For this review, take the finished solid that the model builds, in its own axes (mm). A direction names the side the tool comes from. Give positions to 0.01 mm unless a question says otherwise; leave off trailing zeros. Loops run counter-clockwise (first coordinate to the right, second up) from the corner with the lowest first, then second, coordinate; pieces in that order, holes last. Notation, with made-up numbers: (30.25, 55) - (89.25, 55) arc R20 ccw to (89.25, 67) - close; hole circle Ø9 at (39, 21.5). An arc over 180 degrees is marked (long way). Use CSV: the item, a comma, the result in double quotes. Start each with the question number.
1. For pin 1 (1 mm diameter, centred on x = 765, y = 14, fed in from +Z); pin 2 (9.5 mm diameter, centred on x = 750, y = 29.31, fed in from +Z) (1 decimal); pin 3 (8.5 mm diameter, centred on x = 755.5, y = 37, fed in from -Z); pin 4 (1 mm diameter, centred on x = 767, z = -4, fed in from -Y), all flat-tipped, find the tip position at first contact; note any pin that passes through.
2. Mouldability with a two-part tool opening along Y and no side actions: class faces 1 (the flat face through (750, 15, -10)), 2 (the flat face through (745, 40, 1)) as pulls with the +Y half, pulls with the -Y half, needs draft (parallel to the pull), parting line crosses it, or undercut.
3. For faces 3 (the flat face through (755, 40, 1)), 4 (the flat face through (750, 20, -1)), 5 (the flat face through (750, 20, 3)), list the 3-axis set-ups (+Z, -Z, +X, -X, +Y, -Y) from which the entire face can be reached by the end or side of a thin tool; tool diameter is ignored.
4. Take a section at B-B on x = 750. Give the boundary of the cut face in (y, z), plus the area to 3 significant figures.
5. Take a section at A-A on z = -5. State how many separate pieces and enclosed holes the cut face has, plus the area to 3 significant figures.
6. Wall thickness on line 1 (Y direction, x = 750, z = -3.75); line 2 (Z direction, x = 740, y = 28.5); line 3 (X direction, y = 34.5, z = -2): over which ranges is each line inside the solid? List them lowest first.
```python
from build123d import *

# Parameters (mm, degrees)
SKETCH1_R               = 22.5
BOSS_EXTRUDE1_DEPTH     = 3
SKETCH2_R               = 19.5
BOSS_EXTRUDE2_DEPTH     = 10
SKETCH3_R               = 1.5
CUT_EXTRUDE1_DEPTH      = 13
CUT_EXTRUDE2_DEPTH      = 60.505474974
CUT_EXTRUDE2_DEPTH_BACK = 60.505474974
SKETCH4_R               = 1.5
SKETCH5_R               = 14
CUT_EXTRUDE3_DEPTH      = 9
FILLET1_R               = 3
FILLET2_R               = 2


with BuildPart() as part:
    # Sketch1 → Boss-Extrude1 (new body)
    with BuildSketch(Plane.XY):
        with Locations((750, 29.313623227)):
            Circle(SKETCH1_R)
    extrude(amount=BOSS_EXTRUDE1_DEPTH)

    # Sketch2 → Boss-Extrude2 (add)
    with BuildSketch(Plane(origin=(0, 0, 0), x_dir=(-1, 0, 0), z_dir=(0, 0, -1))):
        with Locations((-750, 29.313623227)):
            Circle(SKETCH2_R)
    extrude(amount=BOSS_EXTRUDE2_DEPTH)

    # Sketch3 → Cut-Extrude1 (cut)
    with BuildSketch(Plane.XY.offset(3)):
        with Locations((761.66726189, 17.646361337)):
            Circle(SKETCH3_R)
        with Locations((738.33273811, 17.646361337)):
            Circle(SKETCH3_R)
        with Locations((738.33273811, 40.980885116)):
            Circle(SKETCH3_R)
        with Locations((761.66726189, 40.980885116)):
            Circle(SKETCH3_R)
        with BuildLine():
            Line((748, 47.313623227), (752, 47.313623227))
            ThreePointArc((752, 47.313623227), (754.121320344, 46.43494357), (755, 44.313623227))
            Line((755, 44.313623227), (755, 35.313623227))
            ThreePointArc((755, 35.313623227), (750, 21.503373551), (745, 35.313623227))
            Line((745, 35.313623227), (745, 44.313623227))
            ThreePointArc((745, 44.313623227), (745.878679656, 46.43494357), (748, 47.313623227))
        make_face()
    extrude(amount=-CUT_EXTRUDE1_DEPTH, mode=Mode.SUBTRACT)

    # Sketch4 → Cut-Extrude2 (cut, two sides: drawn at the far end of the back side and taken through both)
    with BuildSketch(Plane(origin=(745, 0, 0), x_dir=(0, 0, -1), z_dir=(1, 0, 0)).offset(-CUT_EXTRUDE2_DEPTH_BACK)):
        with Locations((5, 29.313623227)):
            Circle(SKETCH4_R)
    extrude(amount=CUT_EXTRUDE2_DEPTH + CUT_EXTRUDE2_DEPTH_BACK, mode=Mode.SUBTRACT)

    # Sketch5 → Cut-Extrude3 (cut)
    with BuildSketch(Plane(origin=(0, 0, -10), x_dir=(-1, 0, 0), z_dir=(0, 0, -1))):
        with Locations((-750, 29.313623227)):
            Circle(SKETCH5_R)
    extrude(amount=-CUT_EXTRUDE3_DEPTH, mode=Mode.SUBTRACT)

    # Fillet1
    fillet1_edges = [part.edges().sort_by_distance(p)[0] for p in [
        (755, 35.313623227, 1),
        (745, 35.313623227, 1),
        (755, 42.390320057, -5.5),
        (745, 42.390320057, -5.5),
    ]]
    fillet(fillet1_edges, radius=FILLET1_R - 0.0001)  # a hair under: the kernel refuses the full size

    # Fillet2
    fillet2_edges = [part.edges().sort_by_distance(p)[0] for p in [
        (727.5, 29.313623227, 3),
    ]]
    fillet(fillet2_edges, radius=FILLET2_R)


solid = part.part
```
Check result:
1,pin 1,"stops at z = 2.95"
1,pin 2,"passes through"
1,pin 3,"stops at z = -1"
1,pin 4,"stops at y = 18.92"
2,face 1,"needs draft"
2,face 2,"undercut"
3,face 3,"+Z, -Z"
3,face 4,"-Z"
3,face 5,"+Z, +X, -X, +Y, -Y"
4,outline,"(6.81, 0) - (9.81, 0) - (9.81, -10) - (15.31, -10) - (15.31, -1) - (21.5, -1) - (21.5, 3) - (8.81, 3) arc R2 ccw to (6.81, 1) - close; (47.31, -10) - (48.81, -10) - (48.81, 0) - (51.81, 0) - (51.81, 1) arc R2 ccw to (49.81, 3) - (47.31, 3) - close"
4,area,"132 mm²"
5,separate pieces,"2"
5,enclosed holes,"4"
5,area,"477 mm²"
6,line 1,"y = 9.81 to 15.31, 47.31 to 48.81"
6,line 2,"z = -1 to 3"
6,line 3,"x = 731.2 to 737, 763 to 768.8"
